CAD build for the part. Positions are in the model's coordinates, mm. A direction names the side the tool comes from. Round coordinates to 2 decimals unless told otherwise and drop trailing zeros. Write each loop counter-clockwise with the first axis right and the second up, starting at its lowest first coordinate (ties: lowest second). Pieces come first, ordered by that corner, then holes. Notation, with made-up numbers: (77.25, 23) - (133.25, 23) arc R16 cw to (133.25, 52) - close; hole circle Ø5 at (59, 31.25). An arc over 180 degrees is marked (long way). Answer in a Markdown table with one row per item.
```python
from build123d import *

# Parameters (mm, degrees)
ESQUISSE1_W             = 8
ESQUISSE1_H             = 36
BOSS_EXTRU_3_DEPTH      = 36
ESQUISSE9_R             = 8.1
ENL_V_MAT_EXTRU_1_DEPTH = 10
BOSS_EXTRU_4_START      = -3
ESQUISSE10_R            = 8.1
ESQUISSE10_R_2          = 4
BOSS_EXTRU_4_DEPTH      = 3
ESQUISSE13_R            = 2
ENL_V_MAT_EXTRU_2_DEPTH = 15
CONG_1_R                = 10


with BuildPart() as part:
    # Esquisse1 → Boss.-Extru.3 (new body)
    with BuildSketch(Plane(origin=(0, 0, 0), x_dir=(1, 0, 0), z_dir=(0, 1, 0))):
        with Locations((4, 18)):
            Rectangle(ESQUISSE1_W, ESQUISSE1_H)
    extrude(amount=BOSS_EXTRU_3_DEPTH)

    # Esquisse9 → Enl_v. mat.-Extru.1 (cut)
    with BuildSketch(Plane(origin=(8, 0, 0), x_dir=(0, 0, -1), z_dir=(1, 0, 0))):
        with Locations((18, 18)):
            Circle(ESQUISSE9_R)
    extrude(amount=-ENL_V_MAT_EXTRU_1_DEPTH, mode=Mode.SUBTRACT)

    # Esquisse10 → Boss.-Extru.4 (add)
    with BuildSketch(Plane.ZY.offset(BOSS_EXTRU_4_START)):
        with Locations(Location((-18, 18, 0), (0, 0, 180))):
            Circle(ESQUISSE10_R)
        with Locations((-18, 18)):
            Circle(ESQUISSE10_R_2, mode=Mode.SUBTRACT)
    extrude(amount=BOSS_EXTRU_4_DEPTH)

    # Esquisse13 → Enl_v. mat.-Extru.2 (cut)
    with BuildSketch(Plane.XZ):
        with Locations(Location((4, -4, 0), (0, 0, 270))):
            Circle(ESQUISSE13_R)
        with Locations(Location((4, -32, 0), (0, 0, 270))):
            Circle(ESQUISSE13_R)
    extrude(amount=-ENL_V_MAT_EXTRU_2_DEPTH, mode=Mode.SUBTRACT)

    # Cong_1
    cong_1_edges = [part.edges().sort_by_distance(p)[0] for p in [
        (4, 36, -36),
        (4, 36, 0),
    ]]
    fillet(cong_1_edges, radius=CONG_1_R)


solid = part.part
```
Q1. Flat gauge pins, fed straight in: pin 1 (2 mm diameter, centred on x = 3.5, z = -31.5, fed in from -Y); pin 2 (3 mm diameter, centred on x = 1, z = -29, fed in from +Y); pin 3 (9.5 mm diameter, centred on y = 18, z = -18, fed in from +X). Where does each tip first touch, or does it go through?
Computed:
| item | result |
|---|---|
| pin 1 | stops at y = 15 |
| pin 2 | stops at y = 35.89 |
| pin 3 | stops at x = 3 |
Q2. Saw through at D-D on z = -4. List the corners of the cut face in (x, y).
Computed:
| item | result |
|---|---|
| outline | (0, 0) - (2, 0) - (2, 15) - (6, 15) - (6, 0) - (8, 0) - (8, 34) - (0, 34) - close |
Q3. Drill centre lines: line 1 (Y direction, x = 6.95, z = -18); line 2 (Y direction, x = 0.6, z = -18); line 3 (X direction, y = 12, z = -4). Where is each one in solid material? Low to high.
Computed:
| item | result |
|---|---|
| line 1 | y = 0 to 9.9, 26.1 to 36 |
| line 2 | y = 0 to 14, 22 to 36 |
| line 3 | x = 0 to 2, 6 to 8 |
Q4. Saw through at A-A on z = -18. List the corners of the cut face in (x, y), then the cut area to 3 significant figures.
Computed:
| item | result |
|---|---|
| outline | (0, 0) - (8, 0) - (8, 9.9) - (3, 9.9) - (3, 14) - (0, 14) - close; (0, 22) - (3, 22) - (3, 26.1) - (8, 26.1) - (8, 36) - (0, 36) - close |
| area | 183 mm2 |
Q5. Saw through at C-C on y = 18. List the corners of the cut face in (x, z), then the cut area to 3 significant figures.
Computed:
| item | result |
|---|---|
| outline | (0, -36) - (8, -36) - (8, -26.1) - (3, -26.1) - (3, -22) - (0, -22) - close; (0, -14) - (3, -14) - (3, -9.9) - (8, -9.9) - (8, 0) - (0, 0) - close |
| area | 183 mm2 |
Q6. 3-axis set-ups, long thin cutter, end or side, ignore diameter. For faces 1 (the cylindrical face through (2.8, 7.4, -2.4)), 2 (the cylindrical face through (4.06, 32.99, -2.85)): which of +Z, -Z, +X, -X, +Y, -Y reach the whole face in a straight line?
Computed:
| item | result |
|---|---|
| face 1 | -Y |
| face 2 | +Z, +X, -X, +Y |
Q7. Saw through at B-B on x = 6.75. List the corners of the cut face in (y, z), then the cut area to 3 significant figures.
Computed:
| item | result |
|---|---|
| outline | (0, -36) - (26, -36) arc R10 ccw to (36, -26) - (36, -10) arc R10 ccw to (26, 0) - (0, 0) - close; hole circle Ø16.2 at (18, -18) |
| area | 1,050 mm2 |
Q8. Pull direction Y, two halves, no side cores. Call faces 3 (the cylindrical face through (5.54, 18.36, -9.91)), 4 (the flat face through (4, 15, -4)), 5 (the flat face through (3, 20, -14)), 6 (the flat face through (4, 36, -18)): released by +Y, released by -Y, zero draft, split by the parting line, or undercut.
Computed:
| item | result |
|---|---|
| face 3 | undercut |
| face 4 | released by -Y |
| face 5 | undercut |
| face 6 | released by +Y |
